from build123d import *

# Parameters (mm, degrees)
SKETCH1_R            = 38.5
BOSS_EXTRUDE1_DEPTH  = 103
BOSS_EXTRUDE2_DEPTH  = 28
CUT_EXTRUDE1_DEPTH   = 28
SHELL2_START         = 4
SHELL2_OUTLINE_R     = 34.5
SHELL2_DEPTH         = 95
SHELL2_START_2       = 107
SHELL2_2_DEPTH       = 24
SHELL2_START_3       = 99
SHELL2_3_OUTLINE_R   = 2
SHELL2_3_DEPTH       = 12.767166294
SHELL2_START_4       = 109.767166294
SHELL2_4_OUTLINE_R   = 7.6
SHELL2_4_OUTLINE_R_2 = 2
SHELL2_4_DEPTH       = 2
SKETCH6_R            = 5
BOSS_EXTRUDE3_DEPTH  = 12


# Read off the part's stored shape, not the designer's step: Shell2
with BuildPart() as part:
    # Sketch1 → Boss-Extrude1 (new body)
    with BuildSketch(Plane.XY):
        Circle(SKETCH1_R)
    extrude(amount=BOSS_EXTRUDE1_DEPTH)

    # Sketch3 → Revolve1 (revolve)
    with BuildSketch(Plane(origin=(0, 0, 0), x_dir=(0, 0, -1), z_dir=(1, 0, 0)), mode=Mode.PRIVATE) as revolve1_sk:
        Polygon((-103, 0), (-103, -6), (-105.767166294, -6), (-105.767166294, -11.6), (-115.767166294, -11.6), (-115.767166294, 0), align=None)
    revolve(revolve1_sk.sketch.rotate(Axis((0, 0, 115.767166294), (0, 0, -1)), 270), axis=Axis((0, 0, 115.767166294), (0, 0, -1)))

    # Sketch4 → Boss-Extrude2 (add)
    with BuildSketch(Plane.XY.offset(103)):
        with BuildLine():
            Line((14.466142326, 17.000326533), (15.115842287, 35.408492088))
            ThreePointArc((15.115842287, 35.408492088), (1.281597128, 38.478663033), (-12.726276266, 36.335821064))
            Line((-12.726276266, 36.335821064), (-13.374025691, 17.982920698))
            Line((-13.374025691, 17.982920698), (0.617262695, 17.48911052))
            Line((0.617262695, 17.48911052), (14.466142326, 17.000326533))
        make_face()
        with BuildLine():
            Line((15.115842287, 35.408492088), (15.453762685, 44.982903362))
            Line((15.453762685, 44.982903362), (-12.386405332, 45.965497528))
            Line((-12.386405332, 45.965497528), (-12.726276266, 36.335821064))
            ThreePointArc((-12.726276266, 36.335821064), (1.281597128, 38.478663033), (15.115842287, 35.408492088))
        make_face()
    extrude(amount=BOSS_EXTRUDE2_DEPTH)

    # Sketch5 → Cut-Extrude1 (cut)
    with BuildSketch(Plane(origin=(-13.991288415, 0.493810179, 0), x_dir=(0, 0, 1), z_dir=(-0.9993777439159626, 0.03527215566762106, 0))):
        Polygon((107, 17.5), (131, 41.5), (131, 17.5), align=None)
    extrude(amount=-CUT_EXTRUDE1_DEPTH, mode=Mode.SUBTRACT)

    # Shell2 outline → Shell2 (cut)
    with BuildSketch(Plane.XY.offset(SHELL2_START)):
        Circle(SHELL2_OUTLINE_R)
    extrude(amount=SHELL2_DEPTH, mode=Mode.SUBTRACT)

    # Shell2 2 outline → Shell2 2 (cut)
    with BuildSketch(Plane.XY.offset(SHELL2_START_2)):
        Polygon((-9.235426092, 21.839343051), (10.609719973, 21.138926131), (11.315163087, 41.126481009), (-8.529982979, 41.826897929), align=None)
    extrude(amount=SHELL2_2_DEPTH, mode=Mode.SUBTRACT)

    # Shell2 3 outline → Shell2 3 (cut)
    with BuildSketch(Plane.XY.offset(SHELL2_START_3)):
        with BuildLine():
            Line((-9.235426092, 21.839343051), (10.609719973, 21.138926131))
            Line((10.609719973, 21.138926131), (11.017527996, 32.693486765))
            ThreePointArc((11.017527996, 32.693486765), (1.142536641, 34.481076115), (-8.82912846, 33.351109286))
            Line((-8.82912846, 33.351109286), (-9.235426092, 21.839343051))
        make_face()
        Circle(SHELL2_3_OUTLINE_R)
    extrude(amount=SHELL2_3_DEPTH, mode=Mode.SUBTRACT)

    # Shell2 4 outline → Shell2 4 (cut)
    with BuildSketch(Plane.XY.offset(SHELL2_START_4)):
        Circle(SHELL2_4_OUTLINE_R)
        Circle(SHELL2_4_OUTLINE_R_2, mode=Mode.SUBTRACT)
    extrude(amount=SHELL2_4_DEPTH, mode=Mode.SUBTRACT)

    # Sketch6 → Boss-Extrude3 (add)
    with BuildSketch(Plane(origin=(0, 0, 0), x_dir=(-1, 0, 0), z_dir=(0, 0, -1))):
        with Locations(Location((0, 0, 0), (0, 0, 180))):
            Circle(SKETCH6_R)
    extrude(amount=BOSS_EXTRUDE3_DEPTH)


solid = part.part
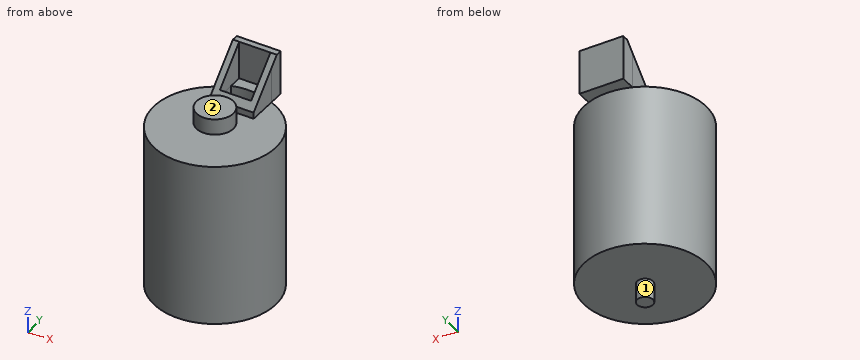
Here's how the part is built. I have some questions about the finished solid (model axes, mm). Face numbers are marked on the shaded views. A direction names the side the tool comes from. Round coordinates to 2 decimals unless told otherwise and drop trailing zeros. Order: outer loops, then holes, each group sorted by start corner. A loop starts at its lowest first (then second) coordinate and runs counter-clockwise, first axis right, second up. Notation, with made-up numbers: M -8,81 L 4,81 A5 cw 4,88 Z; hole C 3.5,33.25 d6. An arc over 180 degrees is marked long. Return JSON: item names as keys, results as strings. Group by question number.
1. On a 3-axis mill with a long thin cutter (end or side, diameter ignored), from which of +Z, -Z, +X, -X, +Y, -Y can I reach the whole of each face in a straight line? I mean the marked faces 1 and 2. Say none if no direction works.
2. I'm going to push flat-ended pins straight in: pin 1 Ø1.5 at (x, z) = (10, 107.5) entering from -Y; pin 2 Ø10 at (x, y) = (18, 15.5) entering from +Z; pin 3 Ø12 at (x, y) = (1.5, -0.5) entering from +Z. Where does each tip first touch, or does it pass through?
3. If we section it at C-C on z = 65: List the corners of the cut face in (x, y) for me, then the cut area to 3 significant figures.
4. If we section it at A-A on x = -25: List the corners of the cut face in (y, z) for me.
5. If we section it at D-D on y = 0: List the corners of the cut face in (x, z) for me, then the cut area to 3 significant figures.
6. If we section it at B-B on y = -13.5: List the corners of the cut face in (x, z) for me, then the cut area to 3 significant figures.
7. Please list where these lines run through material, in increasing order: probe 1 along Z at (x, y) = (3, 0.5); probe 2 along Z at (x, y) = (19, 1); probe 3 along X at (y, z) = (0, 54).
Reply:
{
 "1": {"face 1": "-Z", "face 2": "+Z, +X, -X, -Y"},
 "2": {"pin 1": "y = -7", "pin 2": "z = 109.11", "pin 3": "z = 115.77"},
 "3": {"outline": "C 0,0 d77; hole C 0,0 d69", "area": "917 mm^2"},
 "4": {"outline": "M -29.28,0 L 29.28,0 L 29.28,103 L -29.28,103 Z; hole M -23.77,4 L 23.77,4 L 23.77,99 L -23.77,99 Z"},
 "5": {"outline": "M -38.5,0 L -5,0 L -5,-12 L 5,-12 L 5,0 L 38.5,0 L 38.5,103 L 6,103 L 6,105.77 L 11.6,105.77 L 11.6,115.77 L -11.6,115.77 L -11.6,105.77 L -6,105.77 L -6,103 L -38.5,103 Z; hole M -34.5,4 L 34.5,4 L 34.5,99 L 2,99 L 2,109.77 L 7.6,109.77 L 7.6,111.77 L -7.6,111.77 L -7.6,109.77 L -2,109.77 L -2,99 L -34.5,99 Z", "area": "1,690 mm^2"},
 "6": {"outline": "M -36.06,0 L 36.06,0 L 36.06,103 L -36.06,103 Z; hole M -31.75,4 L 31.75,4 L 31.75,99 L -31.75,99 Z", "area": "1,400 mm^2"},
 "7": {"probe 1": "-12 to 4, 99 to 109.77, 111.77 to 115.77", "probe 2": "0 to 4, 99 to 103", "probe 3": "-38.5 to -34.5, 34.5 to 38.5"}
}
